Source: CAD feature listing. Evaluate the final solid. Frame: model axes, mm. Face numbers are marked on the shaded views. A direction names the side the tool comes from. Round coordinates to 2 decimals unless told otherwise and drop trailing zeros. Loops run counter-clockwise (first coordinate to the right, second up) from the corner with the lowest first, then second, coordinate; pieces in that order, holes last. Notation, with made-up numbers: M 62,-9.75 L 99,-9.75 A20 cw 99,3.25 Z; hole C 42.5,61.25 d7. An arc over 180 degrees is marked long. One line per item, written item: value.
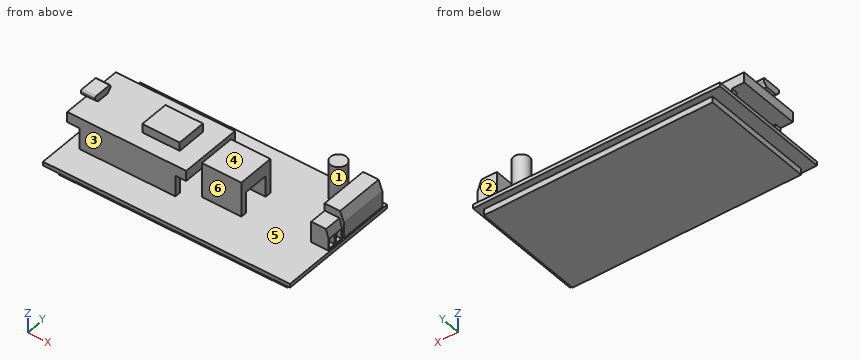
from build123d import *

# Parameters (mm, degrees)
F0_W      = 100
F0_H      = 50.5
F1_DEPTH  = 1.6
F2_W      = 7.8
F2_H      = 20
F3_DEPTH  = 10.5
F4_SIZE2  = 1.5
F4_SIZE   = 4
F2_W_2    = 7
F2_H_2    = 7
F5_DEPTH  = 8.5
F6_SIZE2  = 1
F6_SIZE   = 3.5
F2_R      = 3.25
F7_DEPTH  = 15
F2_W_3    = 38.8
F2_H_3    = 2.5
F2_W_4    = 16
F8_DEPTH  = 8.6
F9_W      = 92.5
F9_H      = 46.1
F10_DEPTH = 2.5
F11_W     = 2.9
F11_H     = 4
F12_DEPTH = 2
F13_W     = 16
F13_H     = 15.1
F14_DEPTH = 5.5
F15_W     = 48.2
F15_H     = 25.3
F16_DEPTH = 4.2
F17_W     = 15.16
F17_H     = 12.06
F18_DEPTH = 3.5
F19_W     = 5.7
F19_H     = 7.9
F20_DEPTH = 2.9
F22_DEPTH = 5.7
F23_R     = 0.5


with BuildPart() as f1:
    # F0 (on Top) → F1 (new body)
    with BuildSketch(Plane.XY):
        Rectangle(F0_W, F0_H)
    extrude(amount=F1_DEPTH)

    # F2 (on face) → F3 (join)
    with BuildSketch(Plane.XY.offset(1.6)):
        with Locations((45.6, 13.45)):
            Rectangle(F2_W, F2_H)
    extrude(amount=F3_DEPTH)

    # F4
    f4_edges = [f1.edges().sort_by_distance(p)[0] for p in [
        (49.5, 13.45, 12.1),
    ]]
    f4_side = f1.faces().sort_by_distance((49.5, 13.45, 6.85))[0]
    chamfer(f4_edges, length=F4_SIZE, length2=F4_SIZE2, reference=f4_side)

    # F2 (on face) → F5 (join)
    with BuildSketch(Plane.XY.offset(1.6)):
        with Locations((46, -1.05)):
            Rectangle(F2_W_2, F2_H_2)
    extrude(amount=F5_DEPTH)

    # F6
    f6_edges = [f1.edges().sort_by_distance(p)[0] for p in [
        (49.5, -1.05, 10.1),
    ]]
    f6_side = f1.faces().sort_by_distance((49.5, -1.05, 5.85))[0]
    chamfer(f6_edges, length=F6_SIZE, length2=F6_SIZE2, reference=f6_side)

    # F2 (on face) → F7 (join)
    with BuildSketch(Plane.XY.offset(1.6)):
        with Locations((35.4, 18.75)):
            Circle(F2_R)
    extrude(amount=F7_DEPTH)

    # F2 (on face) → F8 (join)
    with BuildSketch(Plane.XY.offset(1.6)):
        with Locations((-25.3, 11)):
            Rectangle(F2_W_3, F2_H_3)
        with Locations((9, 5.75)):
            Rectangle(F2_W_4, F2_H_3)
        with Locations((9, -6.85)):
            Rectangle(F2_W_4, F2_H_3)
        with Locations((-25.3, -11.8)):
            Rectangle(F2_W_3, F2_H_3)
    extrude(amount=F8_DEPTH)

    # F9 (on face) → F10 (join)
    with BuildSketch(Plane(origin=(0, 0, 0), x_dir=(1, 0, 0), z_dir=(0, 0, -1))):
        with Locations((1.25, 0.3)):
            Rectangle(F9_W, F9_H)
    extrude(amount=F10_DEPTH)

    # F11 (on face) → F12 (cut)
    with BuildSketch(Plane.YZ.offset(49.5)):
        with Locations((-2.9, 4.3)):
            Rectangle(F11_W, F11_H)
        with Locations((0.7, 4.3)):
            Rectangle(F11_W, F11_H)
    extrude(amount=-F12_DEPTH, mode=Mode.SUBTRACT)

    # F13 (on face) → F14 (join)
    with BuildSketch(Plane.XY.offset(10.2)):
        with Locations((9, -0.55)):
            Rectangle(F13_W, F13_H)
    extrude(amount=F14_DEPTH)

    # F15 (on face) → F16 (join)
    with BuildSketch(Plane.XY.offset(10.2)):
        with Locations((-25.6, -0.4)):
            Rectangle(F15_W, F15_H)
    extrude(amount=F16_DEPTH)

    # F17 (on face) → F18 (join)
    with BuildSketch(Plane.XY.offset(14.4)):
        with Locations((-16.88, -0.38)):
            Rectangle(F17_W, F17_H)
    extrude(amount=F18_DEPTH)

    # F19 (on face) → F20 (join)
    with BuildSketch(Plane.XY.offset(14.4)):
        with Locations((-48, -0.4)):
            Rectangle(F19_W, F19_H)
    extrude(amount=F20_DEPTH)

    # F21 (on face) → F22 (cut, through all)
    with BuildSketch(Plane(origin=(-50.85, 0, 0), x_dir=(0, -1, 0), z_dir=(-1, 0, 0))):
        Polygon((4.35, 14.4), (4.35, 15.8), (2.75, 14.4), align=None)
        Polygon((-3.55, 15.8), (-3.55, 14.4), (-1.95, 14.4), align=None)
    extrude(amount=-F22_DEPTH, mode=Mode.SUBTRACT)

    # F23
    f23_edges = [f1.edges().sort_by_distance(p)[0] for p in [
        (-48, 3.55, 15.8),
        (-48, 3.55, 17.3),
        (-48, -4.35, 17.3),
        (-48, -4.35, 15.8),
    ]]
    fillet(f23_edges, radius=F23_R)


solid = f1.part
1. Section query A-A (x = -36). Return the cut outline in (y, z).
Report:
outline: M -25.25,0 L -23.35,0 L -23.35,-2.5 L 22.75,-2.5 L 22.75,0 L 25.25,0 L 25.25,1.6 L 12.25,1.6 L 12.25,14.4 L -13.05,14.4 L -13.05,1.6 L -25.25,1.6 Z; hole M -10.55,1.6 L 9.75,1.6 L 9.75,10.2 L -10.55,10.2 Z
2. Ray query, line 1 (Z direction, x = 3, y = 0.5); line 2 (Y direction, x = -44, z = 6); line 3 (Z direction, x = -42.5, y = 9.5). Return the intervals inside material, ascending. Write a range as [from, to].
Report:
line 1: z = [-2.5, 1.6], [10.2, 15.7]
line 2: y = [-13.05, -10.55], [9.75, 12.25]
line 3: z = [-2.5, 1.6], [10.2, 14.4]
3. Section query C-C (x = 35.4). Return the cut outline in (y, z).
Report:
outline: M -25.25,0 L -23.35,0 L -23.35,-2.5 L 22.75,-2.5 L 22.75,0 L 25.25,0 L 25.25,1.6 L 22,1.6 L 22,16.6 L 15.5,16.6 L 15.5,1.6 L -25.25,1.6 Z
4. Pull-direction query (X, two-part tool) for the marked faces 1 and 2; classes: released by +X, released by -X, zero draft, split by the parting line, or undercut.
Report:
face 1: undercut
face 2: zero draft
5. Reachability of the marked faces 3, 4, 5 and 6 from +Z, -Z, +X, -X, +Y, -Y: full face, straight path, thin tool, end or side. Return the list, or none.
Report:
face 3: +Z, +X, -X, -Y
face 4: +Z, +X, +Y, -Y
face 5: none
face 6: +Z, +X, -Y
6. Section query D-D (x = -10.5). Return the cut outline in (y, z), and give its area (3 significant figures).
Report:
outline: M -25.25,0 L -23.35,0 L -23.35,-2.5 L 22.75,-2.5 L 22.75,0 L 25.25,0 L 25.25,1.6 L 12.25,1.6 L 12.25,14.4 L 5.65,14.4 L 5.65,17.9 L -6.41,17.9 L -6.41,14.4 L -13.05,14.4 L -13.05,1.6 L -25.25,1.6 Z; hole M -10.55,1.6 L 9.75,1.6 L 9.75,10.2 L -10.55,10.2 Z
area: 388 mm2
7. Pin query (flat end, axial travel): pin 1 (0.6 mm diameter, centred on x = 48, y = 1.5, fed in from -Z); pin 2 (8 mm diameter, centred on y = 18.5, z = 10.5, fed in from -X); pin 3 (1.5 mm diameter, centred on y = -15, z = 1.5, fed in from -X). Return the tip coordinate at first contact, or that it passes through.
Report:
pin 1: stops at z = 0
pin 2: stops at x = 32.15
pin 3: stops at x = -50
8. Section query B-B (y = 20). Return the cut outline in (x, z).
Report:
outline: M -50,0 L -45,0 L -45,-2.5 L 47.5,-2.5 L 47.5,0 L 50,0 L 50,1.6 L 49.5,1.6 L 49.5,8.1 L 48,12.1 L 41.7,12.1 L 41.7,1.6 L 38.4,1.6 L 38.4,16.6 L 32.4,16.6 L 32.4,1.6 L -50,1.6 Z
